The model under review builds one solid part; all positions refer to its coordinate system, in mm. Give positions to 0.01 mm unless a question says otherwise; leave off trailing zeros. Order: outer loops, then holes, each group sorted by start corner. A loop starts at its lowest first (then second) coordinate and runs counter-clockwise, first axis right, second up. Notation, with made-up numbers: (-31.75, -27) - (15.25, -27) arc R23 cw to (15.25, -5) - close; hole circle Ø3 at (31.5, 12). An arc over 180 degrees is marked (long way). Write item = value, one per line. Start each with the question number.
1. We need section A-A, the plane y = 228. Give the boundary of the cut face in (x, z).
2. Wall thickness on probe 1 along Y at (x, z) = (176, 150.45); probe 2 along Y at (x, z) = (153.5, 151.7); probe 3 along X at (y, z) = (230, 153.5): over which ranges is each line inside the solid? List them lowest first.
3. For P1, Ø2.5, axis at x = 129.36, y = -135.6, coming from the -Z side, flat-tipped, find the tip position at first contact; note if it passes through.
4. We need section B-B, the plane x = 156. Give the boundary of the cut face in (y, z).
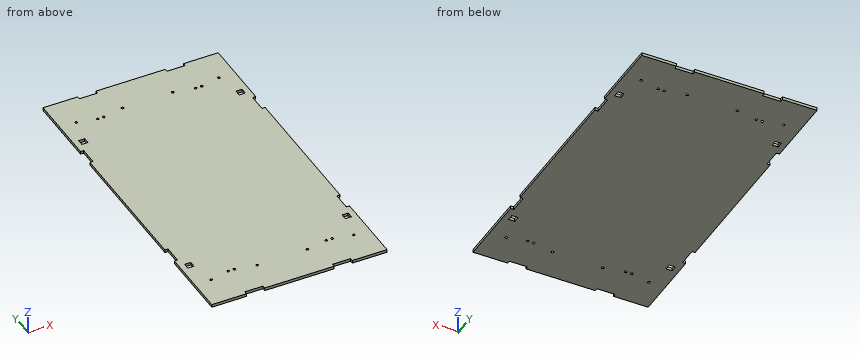
from build123d import *

# Parameters (mm, degrees)
SKETCH1_W           = 300
SKETCH1_H           = 557
SKETCH1_W_2         = 290
SKETCH1_H_2         = 547
BOSS_EXTRUDE1_DEPTH = 150
SKETCH2_W           = 300
SKETCH2_H           = 557
BOSS_EXTRUDE2_DEPTH = 5
SKETCH5_R           = 2.1
CUT_EXTRUDE3_DEPTH  = 10
SKETCH6_W           = 10.5
SKETCH6_H           = 10.5
CUT_EXTRUDE4_DEPTH  = 10
SKETCH8_R           = 1.25
CUT_EXTRUDE6_DEPTH  = 663
SKETCH9_W           = 300
SKETCH9_H           = 557
CUT_EXTRUDE7_DEPTH  = 150
SKETCH10_W          = 31
SKETCH10_H          = 10.8
CUT_EXTRUDE8_DEPTH  = 5
SKETCH13_W          = 10.8
SKETCH13_H          = 31
CUT_EXTRUDE10_DEPTH = 5
SKETCH16_R          = 2.1
CUT_EXTRUDE12_DEPTH = 10


with BuildPart() as part:
    # Sketch1 → Boss-Extrude1 (new body)
    with BuildSketch(Plane.XY):
        with Locations((86.356154307, 86.715846067)):
            Rectangle(SKETCH1_W, SKETCH1_H)
        with Locations((86.356154307, 86.715846067)):
            Rectangle(SKETCH1_W_2, SKETCH1_H_2, mode=Mode.SUBTRACT)
    extrude(amount=BOSS_EXTRUDE1_DEPTH)

    # Sketch2 → Boss-Extrude2 (add)
    with BuildSketch(Plane.XY.offset(150)):
        with Locations((86.356154307, 86.715846067)):
            Rectangle(SKETCH2_W, SKETCH2_H)
    extrude(amount=BOSS_EXTRUDE2_DEPTH)

    # Sketch5 → Cut-Extrude3 (cut)
    with BuildSketch(Plane.XY.offset(155)):
        with Locations((7.766154307, 302.101499848)):
            Circle(SKETCH5_R)
        with Locations((-2.643845693, 302.101499848)):
            Circle(SKETCH5_R)
        with Locations((175.356154307, 302.101499848)):
            Circle(SKETCH5_R)
        with Locations((164.946154307, 302.101499848)):
            Circle(SKETCH5_R)
        with Locations((-2.643845693, -128.669807714)):
            Circle(SKETCH5_R)
        with Locations((7.766154307, -128.669807714)):
            Circle(SKETCH5_R)
        with Locations((164.946154307, -128.669807714)):
            Circle(SKETCH5_R)
        with Locations((175.356154307, -128.669807714)):
            Circle(SKETCH5_R)
    extrude(amount=-CUT_EXTRUDE3_DEPTH, mode=Mode.SUBTRACT)

    # Sketch6 → Cut-Extrude4 (cut)
    with BuildSketch(Plane.XY.offset(155)):
        with Locations((-48.393845693, 261.715846067)):
            Rectangle(SKETCH6_W, SKETCH6_H)
        with Locations((221.106154307, 261.715846067)):
            Rectangle(SKETCH6_W, SKETCH6_H)
        with Locations((221.106154307, -88.284153933)):
            Rectangle(SKETCH6_W, SKETCH6_H)
        with Locations((-48.393845693, -88.284153933)):
            Rectangle(SKETCH6_W, SKETCH6_H)
    extrude(amount=-CUT_EXTRUDE4_DEPTH, mode=Mode.SUBTRACT)

    # Sketch8 → Cut-Extrude6 (cut)
    with BuildSketch(Plane.XZ.offset(191.784153933)):
        with Locations(Location((91.506154307, 9.8, 0), (0, 0, 270))):
            Circle(SKETCH8_R)
        with Locations(Location((81.206154307, 9.8, 0), (0, 0, 270))):
            Circle(SKETCH8_R)
    extrude(amount=-CUT_EXTRUDE6_DEPTH, mode=Mode.SUBTRACT)

    # Sketch9 → Cut-Extrude7 (cut)
    with BuildSketch(Plane(origin=(0, 0, 0), x_dir=(-1, 0, 0), z_dir=(0, 0, -1))):
        with Locations((-86.356154307, 86.715846067)):
            Rectangle(SKETCH9_W, SKETCH9_H)
    extrude(amount=-CUT_EXTRUDE7_DEPTH, mode=Mode.SUBTRACT)

    # Sketch10 → Cut-Extrude8 (cut)
    with BuildSketch(Plane(origin=(0, 0, 150), x_dir=(-1, 0, 0), z_dir=(0, 0, -1))):
        with Locations((-11.356154307, -191.784153933)):
            Rectangle(SKETCH10_W, SKETCH10_H)
        with Locations((-161.356154307, -191.784153933)):
            Rectangle(SKETCH10_W, SKETCH10_H)
        with Locations((-161.356154307, 365.215846067)):
            Rectangle(SKETCH10_W, SKETCH10_H)
        with Locations((-11.356154307, 365.215846067)):
            Rectangle(SKETCH10_W, SKETCH10_H)
    extrude(amount=-CUT_EXTRUDE8_DEPTH, mode=Mode.SUBTRACT)

    # Sketch13 → Cut-Extrude10 (cut)
    with BuildSketch(Plane(origin=(0, 0, 150), x_dir=(-1, 0, 0), z_dir=(0, 0, -1))):
        with Locations((63.643845693, -52.534153933)):
            Rectangle(SKETCH13_W, SKETCH13_H)
        with Locations((63.643845693, 225.965846067)):
            Rectangle(SKETCH13_W, SKETCH13_H)
        with Locations((-236.356154307, 225.965846067)):
            Rectangle(SKETCH13_W, SKETCH13_H)
        with Locations((-236.356154307, -52.534153933)):
            Rectangle(SKETCH13_W, SKETCH13_H)
    extrude(amount=-CUT_EXTRUDE10_DEPTH, mode=Mode.SUBTRACT)

    # Sketch16 → Cut-Extrude12 (cut)
    with BuildSketch(Plane.XY.offset(155)):
        with Locations((208.356154307, 309.215846067)):
            Circle(SKETCH16_R)
        with Locations((129.356358153, 309.036381593)):
            Circle(SKETCH16_R)
        with Locations(Location((43.355950462, 309.036381593, 0), (0, 0, 180))):
            Circle(SKETCH16_R)
        with Locations(Location((-35.643845693, 309.215846067, 0), (0, 0, 180))):
            Circle(SKETCH16_R)
        with Locations((-35.643845693, -135.784153933)):
            Circle(SKETCH16_R)
        with Locations((43.355950462, -135.604689459)):
            Circle(SKETCH16_R)
        with Locations(Location((129.356358153, -135.604689459, 0), (0, 0, 180))):
            Circle(SKETCH16_R)
        with Locations(Location((208.356154307, -135.784153933, 0), (0, 0, 180))):
            Circle(SKETCH16_R)
    extrude(amount=-CUT_EXTRUDE12_DEPTH, mode=Mode.SUBTRACT)


solid = part.part
Model answer:
q1.outline = (-58.24, 150) - (230.96, 150) - (230.96, 155) - (-58.24, 155) - close
q2.probe_1 = -186.38 to -130.67, -126.67 to 300.1, 304.1 to 359.82
q2.probe_2 = -186.38 to 359.82
q2.probe_3 = -58.24 to 230.96
q3.P1 = through
q4.outline = (-186.38, 150) - (359.82, 150) - (359.82, 155) - (-186.38, 155) - close
